Autodesk Inventor part; units mm, degrees
ref_plane "YZ Plane" through (0, 0, 0) normal (1, 0, 0) x (0, 1, 0)
ref_plane "XZ Plane" through (0, 0, 0) normal (0, 1, 0) x (-1, 0, 0)
ref_plane "XY Plane" through (0, 0, 0) normal (0, 0, 1) x (1, 0, 0)
sketch "Sketch1" plane through (0, 0, 0) normal (0, 0, 1) x (1, 0, 0)
  line L0 (0, 0) -> (0, 3)
  line L1 (0, 3) -> (2, 3)
  line L2 (2, 3) -> (2, 2)
  line L3 (2, 2) -> (12, 2)
  line L4 (12, 2) -> (12, 0)
  line L5 (12, 0) -> (0, 0)
  point P0 (1, 3)
  point P1 (0, 1.5)
  point P2 (2, 2.5)
  dimension "d0" = 6
  dimension "d1" = 4
  dimension "d2" = 12
  dimension "d3" = 2
revolve "Revolution1" add sketch "Sketch1" angle 360 about axis through (12, 0, 0) along (-1, 0, 0)
chamfer "Chamfer1" distance 0.5 angle 45 2 edges at (0, -3, 0) (12, -2, 0)
properties part number "Axle" material "Steel"
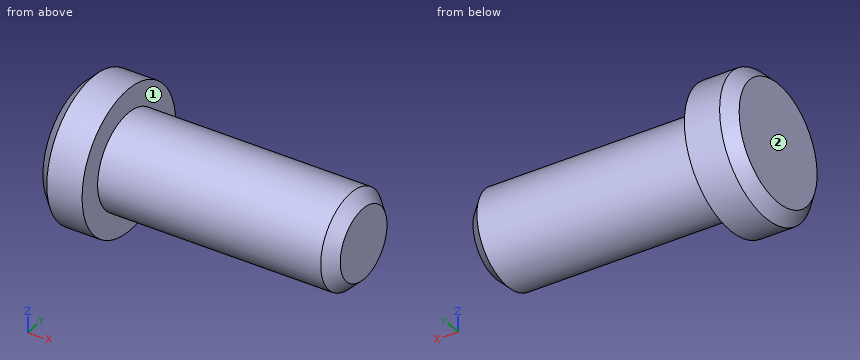
The listing builds one solid part. Answer for the finished solid, in the listing's coordinates (mm). Face numbers are marked on the shaded views. A direction names the side the tool comes from. Round coordinates to 2 decimals unless told otherwise and drop trailing zeros. Order: outer loops, then holes, each group sorted by start corner. A loop starts at its lowest first (then second) coordinate and runs counter-clockwise, first axis right, second up. Notation, with made-up numbers: (56.25, 75) -> (84.25, 75) arc R25 cw to (84.25, 89) -> close; hole circle Ø3 at (30.25, -29.5). An arc over 180 degrees is marked (long way). Write each question's results on one line, items separated by ' | '. Start each with the question number.
Q1. This flat-tipped pin is pushed along its axis until it touches: pin 1 (1.5 mm diameter, centred on x = 7, y = 0.5, fed in from -Z). Where does it stop, or does it pass through?
Q2. Straight lines are drawn through the part: probe 1 along X at (y, z) = (2.3, 0.3); probe 2 along Y at (x, z) = (8, -0.05). For each, find the intervals that lie inside material, in ascending order. Write a range as from..to.
Q3. Find section C-C (x = 11.25). Determine the outline of the cut face in (y, z), then the cut area to 3 significant figures.
Q4. Which of the six approach directions +Z, -Z, +X, -X, +Y, -Y give full straight-line access (tool end or side, diameter ignored) to the marked faces 1 and 2?
Q5. Find section D-D (x = 1.5). Determine the outline of the cut face in (y, z).
Q6. Find section A-A (y = 0). Determine the outline of the cut face in (x, z), then the cut area to 3 significant figures.
Worked answers:
1) pin 1: stops at z = -2
2) probe 1: x = 0..2 | probe 2: y = -2..2
3) outline: circle Ø4 at (0, 0) | area: 12.6 mm2
4) face 1: +X | face 2: +Z, -Z, -X, +Y, -Y
5) outline: circle Ø6 at (0, 0)
6) outline: (0, -2.5) -> (0.5, -3) -> (2, -3) -> (2, -2) -> (11.5, -2) -> (12, -1.5) -> (12, 1.5) -> (11.5, 2) -> (2, 2) -> (2, 3) -> (0.5, 3) -> (0, 2.5) -> close | area: 51.5 mm2
